Could you check a few things on this model? Use its own coordinates, in mm. A direction names the side the tool comes from. Give positions to 0.01 mm unless a question says otherwise; leave off trailing zeros. Loops run counter-clockwise (first coordinate to the right, second up) from the corner with the lowest first, then second, coordinate; pieces in that order, holes last. Notation, with made-up numbers: M -37,-35.5 L 0,-35.5 A24 cw 0,-5.5 Z; hole C -22.75,-33 d1. An arc over 180 degrees is marked long. Use CSV: the item, a comma, the result in double quotes.
Autodesk Inventor part; units mm, degrees
ref_plane "YZ Plane" through (0, 0, 0) normal (1, 0, 0) x (0, 1, 0)
ref_plane "XZ Plane" through (0, 0, 0) normal (0, 1, 0) x (-1, 0, 0)
ref_plane "XY Plane" through (0, 0, 0) normal (0, 0, 1) x (1, 0, 0)
sketch "Эскиз1" plane through (0, 0, 0) normal (0, 0, 1) x (1, 0, 0)
  line L0 (0, 0) -> (0, 30)
  line L1 (3.9, 30) -> (8.5, 30)
  line L2 (8.5, 30) -> (13, 0)
  line L3 (0, 0) -> (13, 0)
  line L4 (3.9, 30) -> (3.9, 10)
  line L5 (3.9, 10) -> (2, 10)
  line L6 (2, 10) -> (2, 0)
  dimension "d0" = 30
  dimension "d1" = 4
  dimension "d2" = 7.8
  dimension "d3" = 17
  dimension "d4" = 26
  dimension "d8" = 10
revolve "Вращение1" add sketch "Эскиз1" angle 360 about axis through (0, 0, 0) along (0, 1, 0)
fillet "Сопряжение1" radius 0.2 1 edges at (-13, 0, 0)
fillet "Сопряжение2" radius 0.5 1 edges at (-8.5, 30, 0)
properties part number "ножки"
1. Please list where these lines run through material, in increasing order: line 1 (X direction, y = 21, z = 0); line 2 (X direction, y = 18.75, z = 0); line 3 (Z direction, x = 0, y = 5.25).
Outcome:
line 1,"-9.85 to -3.9, 3.9 to 9.85"
line 2,"-10.19 to -3.9, 3.9 to 10.19"
line 3,"-12.21 to -2, 2 to 12.21"
2. I'm going to push flat-ended pins straight in: pin 1 Ø3 at (x, y) = (5.5, 20.5) entering from +Z; pin 2 Ø2.5 at (x, z) = (0, 0) entering from +Y; pin 3 Ø12 at (y, z) = (23, -2) entering from -X; pin 4 Ø5 at (x, y) = (5, 18.5) entering from -Z. Where does each tip first touch, or does it pass through?
Outcome:
pin 1,"z = 9.13"
pin 2,"through"
pin 3,"x = -10.41"
pin 4,"z = -10.02"
3. I want a section at D-D, the plane y = 15. List the corners of the cut face in (x, z) for me, then the cut area to 3 significant figures.
Outcome:
outline,"C 0,0 d21.5; hole C 0,0 d7.8"
area,"315 mm2"
4. I want a section at A-A, the plane z = 0. List the corners of the cut face in (x, y) for me, then the cut area to 3 significant figures.
Outcome:
outline,"M -12.97,0.23 A0.2 ccw -12.77,0 L -2,0 L -2,10 L -3.9,10 L -3.9,30 L -8.07,30 A0.5 ccw -8.56,29.57 Z; M 2,0 L 12.77,0 A0.2 ccw 12.97,0.23 L 8.56,29.57 A0.5 ccw 8.07,30 L 3.9,30 L 3.9,10 L 2,10 Z"
area,"449 mm2"
5. If we mould it in two halves opening along X, with no side actions, what happens to faces 1 (the face through (2, 30, -4)), 2 (the face through (0, 5, -2)), 3 (the face through (-2.34, 14.7, -10.54))? For each: +X half, -X half, draft (parallel to the pull), parting line (faces both ways), or undercut.
Outcome:
face 1,"draft"
face 2,"undercut"
face 3,"parting line"
6. I want a section at B-B, the plane x = 0. List the corners of the cut face in (y, z) for me.
Outcome:
outline,"M 0,-12.77 A0.2 ccw 0.23,-12.97 L 29.57,-8.56 A0.5 ccw 30,-8.07 L 30,-3.9 L 10,-3.9 L 10,-2 L 0,-2 Z; M 0,2 L 10,2 L 10,3.9 L 30,3.9 L 30,8.07 A0.5 ccw 29.57,8.56 L 0.23,12.97 A0.2 ccw 0,12.77 Z"
7. Which directions (+Z, -Z, +X, -X, +Y, -Y) give clear straight access to the entire face, cutting with the end or side of a thin tool? Please do faces 4 (the face through (-2, 10, -1)), 5 (the face through (0, 0, 3)).
Outcome:
face 4,"+Y"
face 5,"+Z, -Z, +X, -X, -Y"
8. I want a section at C-C, the plane y = 6. List the corners of the cut face in (x, z) for me, then the cut area to 3 significant figures.
Outcome:
outline,"C 0,0 d24.2; hole C 0,0 d4"
area,"447 mm2"
